Geometry check sheet. Reference: the model listing, model coordinates, mm. A direction names the side the tool comes from. Give positions to 0.01 mm unless a question says otherwise; leave off trailing zeros. Answer as a JSON object with one key per item and string values.
from build123d import *

# Parameters (mm, degrees)
BOSS_EXTRUDE1_DEPTH = 94
FILLET1_R           = 1
CUT_EXTRUDE1_DEPTH  = 95
FILLET2_R           = 0.5
FILLET3_R           = 0.25


with BuildPart() as part:
    # Sketch3 → Boss-Extrude1 (new body)
    with BuildSketch(Plane(origin=(0, 0, 0), x_dir=(1, 0, 0), z_dir=(0, 1, 0))):
        with BuildLine():
            Line((7, 18.5), (7, 19.5))
            ThreePointArc((7, 19.5), (6.646446609, 19.646446609), (6.5, 20))
            Line((6.5, 20), (0, 20))
            Line((0, 20), (0, 13.5))
            ThreePointArc((0, 13.5), (0.353553391, 13.353553391), (0.5, 13))
            Line((0.5, 13), (1.5, 13))
            Line((1.5, 13), (1.5, 16))
            Line((1.5, 16), (3, 16))
            Line((3, 16), (5.5, 13.5))
            Line((5.5, 13.5), (5.5, 10.5))
            Line((5.5, 10.5), (6, 10))
            Line((6, 10), (5.5, 9.5))
            Line((5.5, 9.5), (5.5, 6.5))
            Line((5.5, 6.5), (3, 4))
            Line((3, 4), (1.5, 4))
            Line((1.5, 4), (1.5, 7))
            Line((1.5, 7), (0.5, 7))
            ThreePointArc((0.5, 7), (0.353553391, 6.646446609), (0, 6.5))
            Line((0, 6.5), (0, 0))
            Line((0, 0), (6.5, 0))
            ThreePointArc((6.5, 0), (6.646446609, 0.353553391), (7, 0.5))
            Line((7, 0.5), (7, 1.5))
            Line((7, 1.5), (4, 1.5))
            Line((4, 1.5), (4, 3))
            Line((4, 3), (6.5, 5.5))
            Line((6.5, 5.5), (9.5, 5.5))
            Line((9.5, 5.5), (10, 6))
            Line((10, 6), (10.5, 5.5))
            Line((10.5, 5.5), (13.5, 5.5))
            Line((13.5, 5.5), (16, 3))
            Line((16, 3), (16, 1.5))
            Line((16, 1.5), (13, 1.5))
            Line((13, 1.5), (13, 0.5))
            ThreePointArc((13, 0.5), (13.353553391, 0.353553391), (13.5, 0))
            Line((13.5, 0), (20, 0))
            Line((20, 0), (20, 6.5))
            ThreePointArc((20, 6.5), (19.646446609, 6.646446609), (19.5, 7))
            Line((19.5, 7), (18.5, 7))
            Line((18.5, 7), (18.5, 4))
            Line((18.5, 4), (17, 4))
            Line((17, 4), (14.5, 6.5))
            Line((14.5, 6.5), (14.5, 9.5))
            Line((14.5, 9.5), (14, 10))
            Line((14, 10), (14.5, 10.5))
            Line((14.5, 10.5), (14.5, 13.5))
            Line((14.5, 13.5), (17, 16))
            Line((17, 16), (18.5, 16))
            Line((18.5, 16), (18.5, 13))
            Line((18.5, 13), (19.5, 13))
            ThreePointArc((19.5, 13), (19.646446609, 13.353553391), (20, 13.5))
            Line((20, 13.5), (20, 20))
            Line((20, 20), (13.5, 20))
            ThreePointArc((13.5, 20), (13.353553391, 19.646446609), (13, 19.5))
            Line((13, 19.5), (13, 18.5))
            Line((13, 18.5), (16, 18.5))
            Line((16, 18.5), (16, 17))
            Line((16, 17), (13.5, 14.5))
            Line((13.5, 14.5), (10.5, 14.5))
            Line((10.5, 14.5), (10, 14))
            Line((10, 14), (9.5, 14.5))
            Line((9.5, 14.5), (6.5, 14.5))
            Line((6.5, 14.5), (4, 17))
            Line((4, 17), (4, 18.5))
            Line((4, 18.5), (7, 18.5))
        make_face()
    extrude(amount=BOSS_EXTRUDE1_DEPTH)

    # Fillet1
    fillet1_edges = [part.edges().sort_by_distance(p)[0] for p in [
        (20, 47, 0),
        (0, 47, 0),
        (0, 47, -20),
        (20, 47, -20),
    ]]
    fillet(fillet1_edges, radius=FILLET1_R)

    # Sketch4 → Cut-Extrude1 (cut, through all)
    with BuildSketch(Plane(origin=(0, 94, 0), x_dir=(1, 0, 0), z_dir=(0, 1, 0))):
        with BuildLine():
            Line((10, 11), (11.195582496, 12.195582496))
            ThreePointArc((11.195582496, 12.195582496), (10, 12.5), (8.804417504, 12.195582496))
            Line((8.804417504, 12.195582496), (10, 11))
        make_face()
        with BuildLine():
            ThreePointArc((12.195582496, 11.195582496), (11.767766953, 11.767766953), (11.195582496, 12.195582496))
            Line((11.195582496, 12.195582496), (10, 11))
            Line((10, 11), (11, 10))
            Line((11, 10), (12.195582496, 11.195582496))
        make_face()
        with BuildLine():
            Line((9, 10), (10, 11))
            Line((10, 11), (8.804417504, 12.195582496))
            ThreePointArc((8.804417504, 12.195582496), (8.232233047, 11.767766953), (7.804417504, 11.195582496))
            Line((7.804417504, 11.195582496), (9, 10))
        make_face()
        Polygon((11, 10), (10, 11), (9, 10), (10, 9), align=None)
        with BuildLine():
            Line((7.804417504, 8.804417504), (9, 10))
            Line((9, 10), (7.804417504, 11.195582496))
            ThreePointArc((7.804417504, 11.195582496), (7.5, 10), (7.804417504, 8.804417504))
        make_face()
        with BuildLine():
            Line((10, 9), (9, 10))
            Line((9, 10), (7.804417504, 8.804417504))
            ThreePointArc((7.804417504, 8.804417504), (8.232233047, 8.232233047), (8.804417504, 7.804417504))
            Line((8.804417504, 7.804417504), (10, 9))
        make_face()
        with BuildLine():
            Line((11.195582496, 7.804417504), (10, 9))
            Line((10, 9), (8.804417504, 7.804417504))
            ThreePointArc((8.804417504, 7.804417504), (10, 7.5), (11.195582496, 7.804417504))
        make_face()
        with BuildLine():
            Line((12.195582496, 8.804417504), (11, 10))
            Line((11, 10), (10, 9))
            Line((10, 9), (11.195582496, 7.804417504))
            ThreePointArc((11.195582496, 7.804417504), (11.767766953, 8.232233047), (12.195582496, 8.804417504))
        make_face()
        with BuildLine():
            ThreePointArc((12.5, 10), (12.422700584, 10.616864556), (12.195582496, 11.195582496))
            Line((12.195582496, 11.195582496), (11, 10))
            Line((11, 10), (12.195582496, 8.804417504))
            ThreePointArc((12.195582496, 8.804417504), (12.422700584, 9.383135444), (12.5, 10))
        make_face()
        with BuildLine():
            ThreePointArc((8.804417504, 7.804417504), (8.232233047, 8.232233047), (7.804417504, 8.804417504))
            Line((7.804417504, 8.804417504), (7, 8))
            Line((7, 8), (8, 7))
            Line((8, 7), (8.804417504, 7.804417504))
        make_face()
        with BuildLine():
            Line((13, 8), (12.195582496, 8.804417504))
            ThreePointArc((12.195582496, 8.804417504), (11.767766953, 8.232233047), (11.195582496, 7.804417504))
            Line((11.195582496, 7.804417504), (12, 7))
            Line((12, 7), (13, 8))
        make_face()
        with BuildLine():
            Line((13, 12), (12, 13))
            Line((12, 13), (11.195582496, 12.195582496))
            ThreePointArc((11.195582496, 12.195582496), (11.767766953, 11.767766953), (12.195582496, 11.195582496))
            Line((12.195582496, 11.195582496), (13, 12))
        make_face()
        with BuildLine():
            ThreePointArc((7.804417504, 11.195582496), (8.232233047, 11.767766953), (8.804417504, 12.195582496))
            Line((8.804417504, 12.195582496), (8, 13))
            Line((8, 13), (7, 12))
            Line((7, 12), (7.804417504, 11.195582496))
        make_face()
    extrude(amount=-CUT_EXTRUDE1_DEPTH, mode=Mode.SUBTRACT)

    # Fillet2
    fillet2_edges = [part.edges().sort_by_distance(p)[0] for p in [
        (18.5, 47, -13),
        (18.5, 47, -16),
        (14.5, 47, -10.5),
        (14.5, 47, -9.5),
        (18.5, 47, -4),
        (18.5, 47, -7),
        (13, 47, -1.5),
        (16, 47, -1.5),
        (10.5, 47, -5.5),
        (9.5, 47, -5.5),
        (4, 47, -1.5),
        (7, 47, -1.5),
        (1.5, 47, -7),
        (1.5, 47, -4),
        (5.5, 47, -9.5),
        (5.5, 47, -10.5),
        (1.5, 47, -16),
        (1.5, 47, -13),
        (7, 47, -18.5),
        (4, 47, -18.5),
        (9.5, 47, -14.5),
        (10.5, 47, -14.5),
        (16, 47, -18.5),
        (13, 47, -18.5),
    ]]
    fillet(fillet2_edges, radius=FILLET2_R)

    # Fillet3
    fillet3_edges = [part.edges().sort_by_distance(p)[0] for p in [
        (7, 47, -12),
        (8, 47, -13),
        (12, 47, -13),
        (13, 47, -12),
        (13, 47, -8),
        (12, 47, -7),
        (8, 47, -7),
        (7, 47, -8),
    ]]
    fillet(fillet3_edges, radius=FILLET3_R)


solid = part.part
1) Depth check by flat-ended pin: P1, Ø1.5, axis at x = 10, y = 75, coming from the -Z side; P2, Ø1.4, axis at y = 68, z = -12, coming from the +X side. Enter the tip coordinate at first touch or a pass-through.
Geometry check:
{"P1": "stops at z = -14.5", "P2": "stops at x = 14.5"}
2) Material ranges on line 1 along Z through (x, y) = (2.75, 55.5); line 2 along X through (y, z) = (50.5, -18); line 3 along Z through (x, y) = (3.5, 53.5), recorded low to high. Write a range as from..to.
Geometry check:
{"line 1": "z = -20..-16, -4..0", "line 2": "x = 0..4, 16..20", "line 3": "z = -20..-15.5, -4.5..0"}
3) Tool access check on faces 1 (the face through (12, 46, -5.5)), 2 (the face through (20, 46, -4)). Record the directions out of +Z, -Z, +X, -X, +Y, -Y that give a thin tool (end or side, any length) a straight path to the whole face; none if there is none.
Geometry check:
{"face 1": "+Y, -Y", "face 2": "+Z, -Z, +X, +Y, -Y"}
4) Draft check along Z on faces 3 (the face through (14, 94, -8)), 4 (the face through (16, 46, -20)), 5 (the face through (15, 46, -1.5)). Enter one of: pulls with the +Z half, pulls with the -Z half, needs draft (parallel to the pull), parting line crosses it, or undercut.
Geometry check:
{"face 3": "needs draft", "face 4": "pulls with the -Z half", "face 5": "undercut"}
